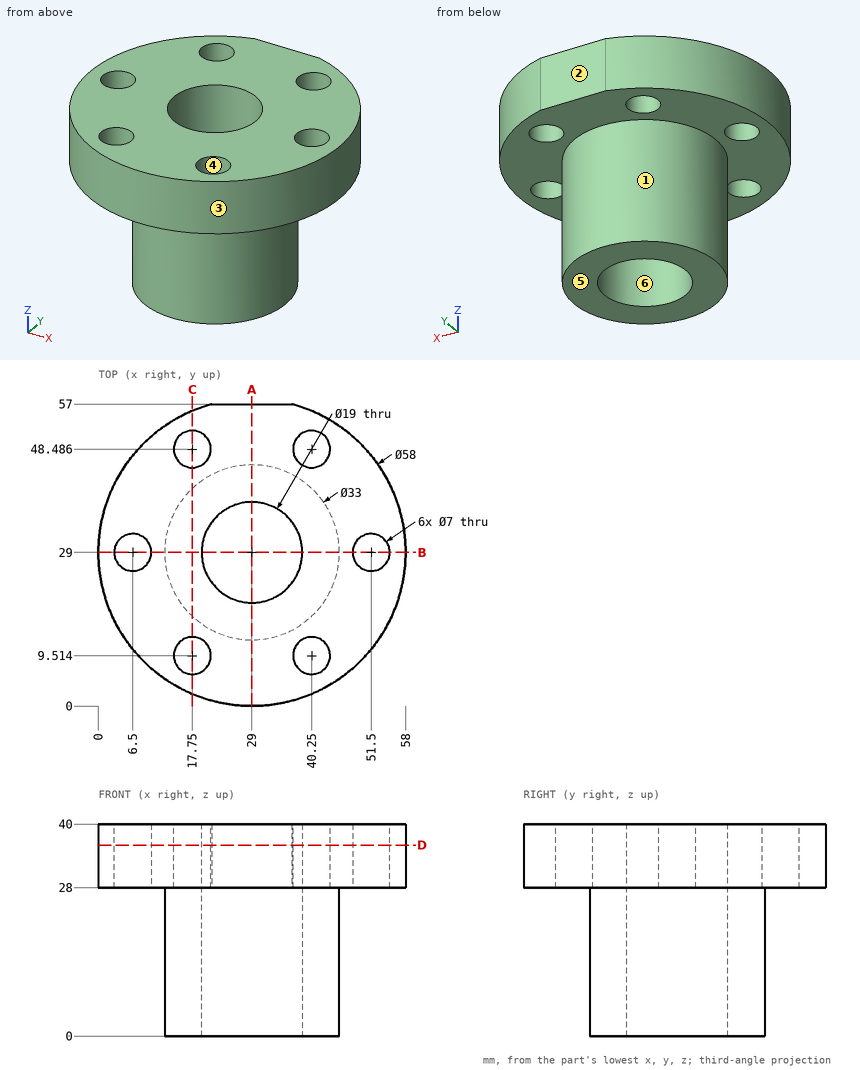
Geometry check sheet. Reference: drawing and pictorial views, mm from the part's lowest x, y, z. A direction names the side the tool comes from. Round coordinates to 2 decimals unless told otherwise and drop trailing zeros. Order: outer loops, then holes, each group sorted by start corner. A loop starts at its lowest first (then second) coordinate and runs counter-clockwise, first axis right, second up. Notation, with made-up numbers: (-0.5, 5) - (12.5, 5) arc R18 ccw to (12.5, 16) - close; hole circle Ø7 at (33, -17). An arc over 180 degrees is marked (long way). One line per question, with ' | ' between items. Start each with the question number.
(1) Sectioned sample at B-B on y = 29. Record the cut outline in (x, z).
(2) Access from +Z, -Z, +X, -X, +Y, -Y to the whole of each face (thin tool, end or side, straight path). Record for the marked faces 1 and 2.
(3) Thickness scan on L1, parallel to X at y = 47, z = 37; L2, parallel to Y at x = 17, z = 33 (1 decimal); L3, parallel to Y at x = 29, z = 2. Record the ranges inside material, lowest first. Write a range as [from, to].
(4) Sectioned sample at C-C on x = 17.75. Record the cut outline in (y, z) (1 decimal), and give its area (3 significant figures).
(5) Release check for a two-part mould opening along X. For the marked faces 3, 4, 5 and 6 record: released by +X, released by -X, zero draft, split by the parting line, or undercut.
(6) Sectioned sample at D-D on z = 36. Count the separate pieces of the cut face and the enclosed holes in it, and give its area (3 significant figures).
(7) Sectioned sample at A-A on x = 29. Record the cut outline in (y, z), and give its area (3 significant figures).
(8) Depth check by flat-ended pin: pin 1 Ø6 at (y, z) = (23.5, 12) entering from +X; pin 2 Ø10 at (x, z) = (31, 11) entering from +Y; pin 3 Ø4 at (x, y) = (17.75, 48.49) entering from -Z; pin 4 Ø10 at (y, z) = (35, 14.5) entering from -X. Enter the tip coordinate at first touch or a pass-through.
Conclusion:
1) outline: (0, 28) - (3, 28) - (3, 40) - (0, 40) - close; (10, 28) - (12.5, 28) - (12.5, 0) - (19.5, 0) - (19.5, 40) - (10, 40) - close; (38.5, 0) - (45.5, 0) - (45.5, 28) - (48, 28) - (48, 40) - (38.5, 40) - close; (55, 28) - (58, 28) - (58, 40) - (55, 40) - close
2) face 1: -Z | face 2: +Z, -Z, +X, -X, +Y
3) L1: x = [6.26, 14.58], [20.92, 37.08], [43.42, 51.74] | L2: y = [2.6, 6.1], [12.9, 45.1], [51.9, 55.4] | L3: y = [12.5, 19.5], [38.5, 45.5]
4) outline: (2.3, 28) - (6, 28) - (6, 40) - (2.3, 40) - close; (13, 28) - (16.9, 28) - (16.9, 0) - (41.1, 0) - (41.1, 28) - (45, 28) - (45, 40) - (13, 40) - close; (52, 28) - (55.7, 28) - (55.7, 40) - (52, 40) - close | area: 1,150 mm2
5) face 3: split by the parting line | face 4: undercut | face 5: zero draft | face 6: undercut
6) separate pieces: 1 | enclosed holes: 7 | area: 2,120 mm2
7) outline: (0, 28) - (12.5, 28) - (12.5, 0) - (19.5, 0) - (19.5, 40) - (0, 40) - close; (38.5, 0) - (45.5, 0) - (45.5, 28) - (57, 28) - (57, 40) - (38.5, 40) - close | area: 848 mm2
8) pin 1: stops at x = 45.31 | pin 2: stops at y = 45.5 | pin 3: passes through | pin 4: stops at x = 12.53
